from build123d import *

# Parameters (mm, degrees)
F0_R          = 60
F1_DEPTH      = 4
F2_DEPTH      = 50
F4_DEPTH      = 566
F5_DEPTH      = 140
F5_DEPTH_BACK = 140
F6_W          = 30
F6_H          = 50
F6_W_2        = 26.8
F6_H_2        = 46.8
F7_DEPTH      = 200


with BuildPart() as f1:
    # F0 (on Top) → F1 (new body)
    with BuildSketch(Plane.XY):
        Polygon((567.5, 55), (567.5, 280), (-567.5, 280), (-567.5, 55), (-562.5, 55), (-562.5, -55), (-567.5, -55), (-567.5, -280), (567.5, -280), (567.5, -55), (562.5, -55), (562.5, 55), align=None)
        with Locations((292.5, 0)):
            Circle(F0_R, mode=Mode.SUBTRACT)
    extrude(amount=F1_DEPTH)

    # F0 (on Top) → F2 (join)
    with BuildSketch(Plane.XY):
        Polygon((-567.5, 280), (567.5, 280), (567.5, 55), (570.5, 55), (570.5, 283), (538.5, 283), (512.5, 283), (13, 283), (-13, 283), (-512.5, 283), (-538.5, 283), (-570.5, 283), (-570.5, 55), (-567.5, 55), align=None)
        Polygon((570.5, -55), (567.5, -55), (567.5, -280), (-567.5, -280), (-567.5, -55), (-570.5, -55), (-570.5, -283), (570.5, -283), align=None)
    extrude(amount=F2_DEPTH)

    # F3 (on face) → F4 (join)
    with BuildSketch(Plane.XZ.offset(283)):
        with BuildLine():
            Line((-512.5, 0), (-538.5, 0))
            ThreePointArc((-538.5, 0), (-539.9142135624, -0.5857864376), (-540.5, -2))
            Line((-540.5, -2), (-540.5, -48))
            ThreePointArc((-540.5, -48), (-539.9142135624, -49.4142135624), (-538.5, -50))
            Line((-538.5, -50), (-512.5, -50))
            ThreePointArc((-512.5, -50), (-511.0857864376, -49.4142135624), (-510.5, -48))
            Line((-510.5, -48), (-510.5, -2))
            ThreePointArc((-510.5, -2), (-511.0857864376, -0.5857864376), (-512.5, 0))
        make_face()
        with BuildLine():
            Line((-538.9, -48), (-538.9, -2))
            ThreePointArc((-538.9, -2), (-538.7828427125, -1.7171572875), (-538.5, -1.6))
            Line((-538.5, -1.6), (-512.5, -1.6))
            ThreePointArc((-512.5, -1.6), (-512.2171572875, -1.7171572875), (-512.1, -2))
            Line((-512.1, -2), (-512.1, -48))
            ThreePointArc((-512.1, -48), (-512.2171572875, -48.2828427125), (-512.5, -48.4))
            Line((-512.5, -48.4), (-538.5, -48.4))
            ThreePointArc((-538.5, -48.4), (-538.7828427125, -48.2828427125), (-538.9, -48))
        make_face(mode=Mode.SUBTRACT)
        with BuildLine():
            Line((13, 0), (-13, 0))
            ThreePointArc((-13, 0), (-14.4142135624, -0.5857864376), (-15, -2))
            Line((-15, -2), (-15, -48))
            ThreePointArc((-15, -48), (-14.4142135624, -49.4142135624), (-13, -50))
            Line((-13, -50), (13, -50))
            ThreePointArc((13, -50), (14.4142135624, -49.4142135624), (15, -48))
            Line((15, -48), (15, -2))
            ThreePointArc((15, -2), (14.4142135624, -0.5857864376), (13, 0))
        make_face()
        with BuildLine():
            Line((-13.4, -48), (-13.4, -2))
            ThreePointArc((-13.4, -2), (-13.2828427125, -1.7171572875), (-13, -1.6))
            Line((-13, -1.6), (13, -1.6))
            ThreePointArc((13, -1.6), (13.2828427125, -1.7171572875), (13.4, -2))
            Line((13.4, -2), (13.4, -48))
            ThreePointArc((13.4, -48), (13.2828427125, -48.2828427125), (13, -48.4))
            Line((13, -48.4), (-13, -48.4))
            ThreePointArc((-13, -48.4), (-13.2828427125, -48.2828427125), (-13.4, -48))
        make_face(mode=Mode.SUBTRACT)
        with BuildLine():
            Line((538.5, 0), (512.5, 0))
            ThreePointArc((512.5, 0), (511.0857864376, -0.5857864376), (510.5, -2))
            Line((510.5, -2), (510.5, -48))
            ThreePointArc((510.5, -48), (511.0857864376, -49.4142135624), (512.5, -50))
            Line((512.5, -50), (538.5, -50))
            ThreePointArc((538.5, -50), (539.9142135624, -49.4142135624), (540.5, -48))
            Line((540.5, -48), (540.5, -2))
            ThreePointArc((540.5, -2), (539.9142135624, -0.5857864376), (538.5, 0))
        make_face()
        with BuildLine():
            ThreePointArc((538.9, -48), (538.7828427125, -48.2828427125), (538.5, -48.4))
            Line((538.5, -48.4), (512.5, -48.4))
            ThreePointArc((512.5, -48.4), (512.2171572875, -48.2828427125), (512.1, -48))
            Line((512.1, -48), (512.1, -2))
            ThreePointArc((512.1, -2), (512.2171572875, -1.7171572875), (512.5, -1.6))
            Line((512.5, -1.6), (538.5, -1.6))
            ThreePointArc((538.5, -1.6), (538.7828427125, -1.7171572875), (538.9, -2))
            Line((538.9, -2), (538.9, -48))
        make_face(mode=Mode.SUBTRACT)
    extrude(amount=-F4_DEPTH)

    # F0 (on Top) → F5 (join, two sides)
    with BuildSketch(Plane.XY) as f5_sk:
        with BuildLine():
            ThreePointArc((-540.5, 285), (-539.9142135624, 283.5857864376), (-538.5, 283))
            Line((-538.5, 283), (-512.5, 283))
            ThreePointArc((-512.5, 283), (-511.0857864376, 283.5857864376), (-510.5, 285))
            Line((-510.5, 285), (-510.5, 311))
            ThreePointArc((-510.5, 311), (-511.0857864376, 312.4142135624), (-512.5, 313))
            Line((-512.5, 313), (-538.5, 313))
            ThreePointArc((-538.5, 313), (-539.9142135624, 312.4142135624), (-540.5, 311))
            Line((-540.5, 311), (-540.5, 285))
        make_face()
        with BuildLine():
            ThreePointArc((-536.9, 284.6), (-538.3142135624, 285.1857864376), (-538.9, 286.6))
            Line((-538.9, 286.6), (-538.9, 309.4))
            ThreePointArc((-538.9, 309.4), (-538.3142135624, 310.8142135624), (-536.9, 311.4))
            Line((-536.9, 311.4), (-514.1, 311.4))
            ThreePointArc((-514.1, 311.4), (-512.6857864376, 310.8142135624), (-512.1, 309.4))
            Line((-512.1, 309.4), (-512.1, 286.6))
            ThreePointArc((-512.1, 286.6), (-512.6857864376, 285.1857864376), (-514.1, 284.6))
            Line((-514.1, 284.6), (-536.9, 284.6))
        make_face(mode=Mode.SUBTRACT)
        with BuildLine():
            Line((-13, 283), (13, 283))
            ThreePointArc((13, 283), (14.4142135624, 283.5857864376), (15, 285))
            Line((15, 285), (15, 311))
            ThreePointArc((15, 311), (14.4142135624, 312.4142135624), (13, 313))
            Line((13, 313), (-13, 313))
            ThreePointArc((-13, 313), (-14.4142135624, 312.4142135624), (-15, 311))
            Line((-15, 311), (-15, 285))
            ThreePointArc((-15, 285), (-14.4142135624, 283.5857864376), (-13, 283))
        make_face()
        with BuildLine():
            Line((13.4, 309.4), (13.4, 286.6))
            ThreePointArc((13.4, 286.6), (12.8142135624, 285.1857864376), (11.4, 284.6))
            Line((11.4, 284.6), (-11.4, 284.6))
            ThreePointArc((-11.4, 284.6), (-12.8142135624, 285.1857864376), (-13.4, 286.6))
            Line((-13.4, 286.6), (-13.4, 309.4))
            ThreePointArc((-13.4, 309.4), (-12.8142135624, 310.8142135624), (-11.4, 311.4))
            Line((-11.4, 311.4), (11.4, 311.4))
            ThreePointArc((11.4, 311.4), (12.8142135624, 310.8142135624), (13.4, 309.4))
        make_face(mode=Mode.SUBTRACT)
        with BuildLine():
            Line((512.5, 283), (538.5, 283))
            ThreePointArc((538.5, 283), (539.9142135624, 283.5857864376), (540.5, 285))
            Line((540.5, 285), (540.5, 311))
            ThreePointArc((540.5, 311), (539.9142135624, 312.4142135624), (538.5, 313))
            Line((538.5, 313), (512.5, 313))
            ThreePointArc((512.5, 313), (511.0857864376, 312.4142135624), (510.5, 311))
            Line((510.5, 311), (510.5, 285))
            ThreePointArc((510.5, 285), (511.0857864376, 283.5857864376), (512.5, 283))
        make_face()
        with BuildLine():
            Line((514.1, 311.4), (536.9, 311.4))
            ThreePointArc((536.9, 311.4), (538.3142135624, 310.8142135624), (538.9, 309.4))
            Line((538.9, 309.4), (538.9, 286.6))
            ThreePointArc((538.9, 286.6), (538.3142135624, 285.1857864376), (536.9, 284.6))
            Line((536.9, 284.6), (514.1, 284.6))
            ThreePointArc((514.1, 284.6), (512.6857864376, 285.1857864376), (512.1, 286.6))
            Line((512.1, 286.6), (512.1, 309.4))
            ThreePointArc((512.1, 309.4), (512.6857864376, 310.8142135624), (514.1, 311.4))
        make_face(mode=Mode.SUBTRACT)
    extrude(amount=-F5_DEPTH)
    extrude(f5_sk.sketch, amount=F5_DEPTH_BACK)

    # F6 (on face) → F7 (join)
    with BuildSketch(Plane(origin=(0, 0, -50), x_dir=(1, 0, 0), z_dir=(0, 0, -1))):
        with Locations((0, 258)):
            Rectangle(F6_W, F6_H)
        with Locations((0, 258)):
            Rectangle(F6_W_2, F6_H_2, mode=Mode.SUBTRACT)
        with Locations((-525.5, 258)):
            Rectangle(F6_W, F6_H)
        with Locations((-525.5, 258)):
            Rectangle(F6_W_2, F6_H_2, mode=Mode.SUBTRACT)
        with Locations((525.5, 258)):
            Rectangle(F6_W, F6_H)
        with Locations((525.5, 258)):
            Rectangle(F6_W_2, F6_H_2, mode=Mode.SUBTRACT)
    extrude(amount=F7_DEPTH)


solid = f1.part
Model file for the job. Use its own axes, mm. A direction names the side the tool comes from. Give positions to 0.01 mm unless a question says otherwise; leave off trailing zeros. Order: outer loops, then holes, each group sorted by start corner. A loop starts at its lowest first (then second) coordinate and runs counter-clockwise, first axis right, second up. Notation, with made-up numbers: M 53,18 L 79,18 A17 cw 79,33 Z; hole C 34.25,-16 d11. An arc over 180 degrees is marked long. Put each result on its own line as item: value. Start each with the question number.
(1) Tool access for faces 1 (the face through (567.5, -166, 27)), 2 (the face through (15, -258, -149)), 3 (the face through (0, -233, -149)): list every direction of +Z, -Z, +X, -X, +Y, -Y with a clear straight run to the whole face (end or side of a thin tool).
(2) Band-saw the part on A-A on z = -163.5. Give the cut face in (x, y), then the cut area to 3 significant figures.
(3) Drill centre lines: L1, parallel to Y at x = 292.5, z = 0.8; L2, parallel to X at y = 119.5, z = 7; L3, parallel to Z at x = -244, y = 27.5. Where is each one in solid material? Low to high. Write a range as [from, to].
(4) Band-saw the part on B-B on y = 0. Count the separate pieces of the cut face and the enclosed holes in it, then the cut area to 3 significant figures.
(5) Band-saw the part on C-C on x = 292.5. Give the cut face in (y, z), then the cut area to 3 significant figures.
(6) Pull direction Z, two halves, no side cores. Call faces 4 (the face through (512.1, -4, -25)), 5 (the face through (511, -256, -250)), 6 (the face through (-510.5, -4, -25)): released by +Z, released by -Z, zero draft, split by the parting line, or undercut.
(7) Pin check, flat tips, straight feed: pin 1 Ø0.6 at (x, y) = (14, -245.5) entering from +Z; pin 2 Ø5 at (x, y) = (418, 1) entering from -Z; pin 3 Ø11.5 at (y, z) = (301, 67.5) entering from +X; pin 4 Ø8 at (x, z) = (-393, -7) entering from -Y. Stop position of each tip, or through.
Results below:
1. face 1: +Z
1. face 2: -Z, +Y, -Y
1. face 3: -Z, +X, -X
2. outline: M -540.5,-283 L -510.5,-283 L -510.5,-233 L -540.5,-233 Z; M -15,-283 L 15,-283 L 15,-233 L -15,-233 Z; M 510.5,-283 L 540.5,-283 L 540.5,-233 L 510.5,-233 Z; hole M -538.9,-281.4 L -512.1,-281.4 L -512.1,-234.6 L -538.9,-234.6 Z; hole M -13.4,-281.4 L 13.4,-281.4 L 13.4,-234.6 L -13.4,-234.6 Z; hole M 512.1,-281.4 L 538.9,-281.4 L 538.9,-234.6 L 512.1,-234.6 Z
2. area: 737 mm2
3. L1: y = [-283, -60], [60, 283]
3. L2: x = [-570.5, -567.5], [567.5, 570.5]
3. L3: z = [0, 4]
4. separate pieces: 2
4. enclosed holes: 3
4. area: 4,750 mm2
5. outline: M -283,0 L -60,0 L -60,4 L -280,4 L -280,50 L -283,50 Z; M 60,0 L 283,0 L 283,50 L 280,50 L 280,4 L 60,4 Z
5. area: 2,060 mm2
6. face 4: undercut
6. face 5: released by -Z
6. face 6: zero draft
7. pin 1: stops at z = 4
7. pin 2: stops at z = 0
7. pin 3: stops at x = 540.5
7. pin 4: passes through
